Work out the finished part from the listing and answer in its coordinate system (mm). Face numbers are marked on the shaded views. Coordinates: 2 decimals unless noted, no trailing zeros. Order: outer loops, then holes, each group sorted by start corner. A loop starts at its lowest first (then second) coordinate and runs counter-clockwise, first axis right, second up. Notation, with made-up numbers: M 17.5,66.5 L 26.5,66.5 A21 cw 26.5,91.5 Z; hole C 78.5,40 d6. An arc over 180 degrees is marked long. Answer in a Markdown table with one row per item. Add a question column.
Item 1: Consider line 1 (X direction, y = -18, z = 3.5); line 2 (Z direction, x = 113.5, y = -1.5). Determine where each line is inside the solid, lowest interval first. Write a range as from..to.
Item 2: The part is cut by section A-A (y = -4). Write down the section's boundary in (x, z).
Item 3: The part is cut by section C-C (z = 22.75). Write down the section's boundary in (x, y).
Item 4: The part is cut by section B-B (x = 10.5). Write down the section's boundary in (y, z).
Item 5: The mould has two halves that part along X. Classify the marked faces 1, 2 and 3: released by +X, released by -X, zero draft, split by the parting line, or undercut.
Item 6: Flat-ended cylindrical pins translate along their axes: pin 1 Ø5 at (x, y) = (83.5, -16.5) entering from +Z; pin 2 Ø10 at (x, z) = (102.5, 10) entering from +Y. Find the tip coordinate at first contact, or state that the pin passes through.
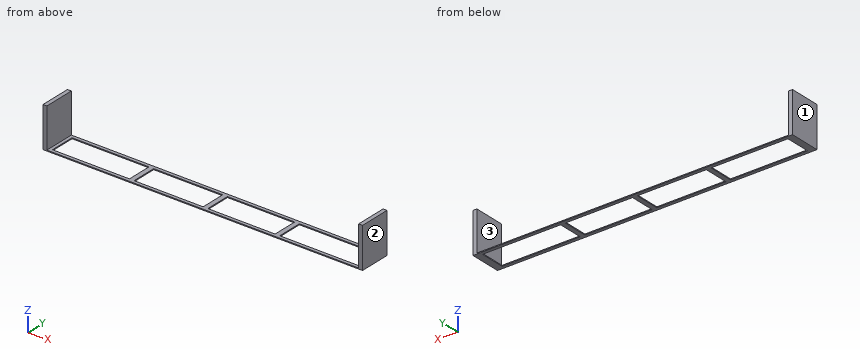
from build123d import *

# Parameters (mm, degrees)
F0_W     = 200
F0_H     = 20
F1_DEPTH = 0.6
F3_W     = 2.5
F3_H     = 20
F4_DEPTH = 26
F2_W     = 49.387012
F2_H     = 16
F2_W_2   = 44.316895
F2_H_2   = 16.031951
F2_W_3   = 43.155649
F2_W_4   = 50.140444
F5_DEPTH = 25


with BuildPart() as f1:
    # F0 (on Top) → F1 (new body)
    with BuildSketch(Plane.XY):
        with Locations((47.677944, -10)):
            Rectangle(F0_W, F0_H)
    extrude(amount=F1_DEPTH)

    # F3 (on Top) → F4 (join)
    with BuildSketch(Plane.XY):
        with Locations((-53.572056, -10)):
            Rectangle(F3_W, F3_H)
        with Locations((148.927944, -10)):
            Rectangle(F3_W, F3_H)
    extrude(amount=F4_DEPTH)

    # F2 (on face) → F5 (cut)
    with BuildSketch(Plane.XY.offset(0.6)):
        with Locations((-25.62855, -10)):
            Rectangle(F2_W, F2_H)
        with Locations((24.223403, -10.015975)):
            Rectangle(F2_W_2, F2_H_2)
        with Locations((70.959676, -10.015975)):
            Rectangle(F2_W_3, F2_H_2)
        with Locations((120.607722, -10)):
            Rectangle(F2_W_4, F2_H)
    extrude(amount=-F5_DEPTH, mode=Mode.SUBTRACT)


solid = f1.part
Reply:
| question | item | result |
|---|---|---|
| 1 | line 1 | x = -54.82..-52.32, 147.68..150.18 |
| 1 | line 2 | z = 0..0.6 |
| 2 | outline | M -54.82,0 L -50.32,0 L -50.32,0.6 L -52.32,0.6 L -52.32,26 L -54.82,26 Z; M -0.94,0 L 2.06,0 L 2.06,0.6 L -0.94,0.6 Z; M 46.38,0 L 49.38,0 L 49.38,0.6 L 46.38,0.6 Z; M 92.54,0 L 95.54,0 L 95.54,0.6 L 92.54,0.6 Z; M 145.68,0 L 150.18,0 L 150.18,26 L 147.68,26 L 147.68,0.6 L 145.68,0.6 Z |
| 3 | outline | M -54.82,-20 L -52.32,-20 L -52.32,0 L -54.82,0 Z; M 147.68,-20 L 150.18,-20 L 150.18,0 L 147.68,0 Z |
| 4 | outline | M -20,0 L -18.03,0 L -18.03,0.6 L -20,0.6 Z; M -2,0 L 0,0 L 0,0.6 L -2,0.6 Z |
| 5 | face 1 | released by -X |
| 5 | face 2 | released by +X |
| 5 | face 3 | undercut |
| 6 | pin 1 | stops at z = 0.6 |
| 6 | pin 2 | passes through |
